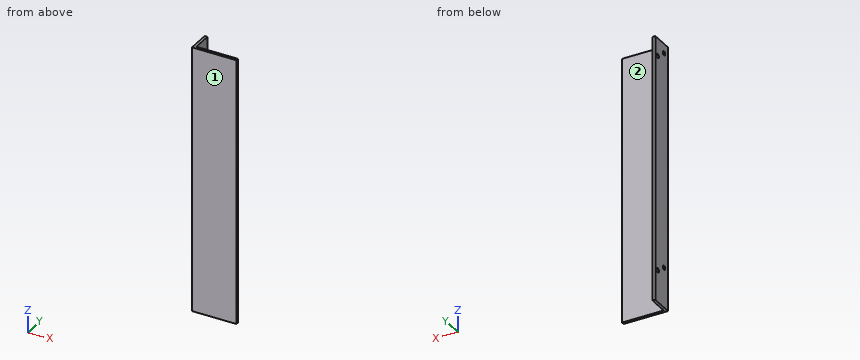
from build123d import *

# Parameters (mm, degrees)
BOSS_EXTRUDE1_DEPTH = 304.8
CUT_EXTRUDE1_REACH  = 312.047
SKETCH2_R           = 2.413


with BuildPart() as part:
    # Sketch1 → Boss-Extrude1 (new body)
    with BuildSketch(Plane.XY):
        Polygon((3.175, 3.175), (3.175, 25.4), (0, 25.4), (0, 0), (50.8, 0), (50.8, 3.175), align=None)
    extrude(amount=BOSS_EXTRUDE1_DEPTH)

    # Sketch2 → Cut-Extrude1 (cut, up to next)
    with BuildSketch(Plane.ZY, mode=Mode.PRIVATE) as cut_extrude1_sk1:
        with Locations((36.5125, 20.6375)):
            Circle(SKETCH2_R)
    cut_extrude1_tool1 = extrude(cut_extrude1_sk1.sketch, amount=-CUT_EXTRUDE1_REACH, mode=Mode.PRIVATE) & part.part
    # Sketch2 → Cut-Extrude1 (cut, up to next)
    with BuildSketch(Plane.ZY, mode=Mode.PRIVATE) as cut_extrude1_sk2:
        with Locations((46.0375, 7.9375)):
            Circle(SKETCH2_R)
    cut_extrude1_tool2 = extrude(cut_extrude1_sk2.sketch, amount=-CUT_EXTRUDE1_REACH, mode=Mode.PRIVATE) & part.part
    # Sketch2 → Cut-Extrude1 (cut, up to next)
    with BuildSketch(Plane.ZY, mode=Mode.PRIVATE) as cut_extrude1_sk3:
        with Locations((284.1625, 20.6375)):
            Circle(SKETCH2_R)
    cut_extrude1_tool3 = extrude(cut_extrude1_sk3.sketch, amount=-CUT_EXTRUDE1_REACH, mode=Mode.PRIVATE) & part.part
    # Sketch2 → Cut-Extrude1 (cut, up to next)
    with BuildSketch(Plane.ZY, mode=Mode.PRIVATE) as cut_extrude1_sk4:
        with Locations((293.6875, 7.9375)):
            Circle(SKETCH2_R)
    cut_extrude1_tool4 = extrude(cut_extrude1_sk4.sketch, amount=-CUT_EXTRUDE1_REACH, mode=Mode.PRIVATE) & part.part
    add(cut_extrude1_tool1.solids().sort_by_distance((0, 20.6375, 36.5125))[0], mode=Mode.SUBTRACT)
    add(cut_extrude1_tool2.solids().sort_by_distance((0, 7.9375, 46.0375))[0], mode=Mode.SUBTRACT)
    add(cut_extrude1_tool3.solids().sort_by_distance((0, 20.6375, 284.1625))[0], mode=Mode.SUBTRACT)
    add(cut_extrude1_tool4.solids().sort_by_distance((0, 7.9375, 293.6875))[0], mode=Mode.SUBTRACT)


solid = part.part
Can you work these out from the model? Positions are in its coordinate system, mm. Face numbers are marked on the shaded views. A direction names the side the tool comes from. Coordinates: 2 decimals unless noted, no trailing zeros. Write each loop counter-clockwise with the first axis right and the second up, starting at its lowest first coordinate (ties: lowest second). Pieces come first, ordered by that corner, then holes.
Q1. Imagine slicing it at A-A, the plane z = 252. List the corners of the cut face in (x, y) for me (3 decimals), plus the area to 3 significant figures.
Results found:
outline: (0, 0) - (50.8, 0) - (50.8, 3.175) - (3.175, 3.175) - (3.175, 25.4) - (0, 25.4) - close
area: 232 mm2
Q2. Which directions (+Z, -Z, +X, -X, +Y, -Y) give clear straight access to the entire face, cutting with the end or side of a thin tool? Please do the marked faces 1 and 2.
Results found:
face 1: +Z, -Z, +X, -X, -Y
face 2: +Z, -Z, +X, +Y
Q3. Imagine slicing it at B-B, the plane y = 13.25. List the corners of the cut face in (x, z) for me (3 decimals).
Results found:
outline: (0, 0) - (3.175, 0) - (3.175, 304.8) - (0, 304.8) - close
Q4. Please list where this line runs through material, in increasing order: L1, parallel to Y at x = 11.5, z = 228 (3 decimals).
Results found:
L1: y = 0 to 3.175
Q5. For P1, Ø12, axis at y = 21.5, z = 71.5, coming from the +X side (3 decimals); P2, Ø3, axis at y = 4, z = 185, coming from the -X side; P3, Ø5, axis at x = 24, z = 228, coming from the +Y side (3 decimals), each with a flat end and sliding along its axis, tell me the tip position at first contact or that it passes through.
Results found:
P1: stops at x = 3.175
P2: stops at x = 0
P3: stops at y = 3.175
